Part model, mm, in its own coordinate system. Round coordinates to 2 decimals unless told otherwise and drop trailing zeros. Loops run counter-clockwise (first coordinate to the right, second up) from the corner with the lowest first, then second, coordinate; pieces in that order, holes last.
(1) Flat gauge pins, fed straight in: pin 1 (0.8 mm diameter, centred on y = 1.5, z = -2.5, fed in from -X); pin 2 (1.8 mm diameter, centred on x = -43.25, z = -31.5, fed in from +Y). Where does each tip first touch, or does it go through?
(2) Probe probe 1 along Z at (x, y) = (22, 2.3); probe 2 along X at (y, z) = (1.9, -31.5); probe 3 along Z at (x, y) = (-41, 2.75). List the from-to ranges inside material, lowest first.
(3) Cut at B-B on z = -6.5. List the corners of the cut face in (x, y), then the cut area to 4 significant figures.
(4) Cut at C-C on y = 0.6. Count the separate pieces of the cut face and the enclosed holes in it, then the cut area to 3 significant figures.
(5) Cut at A-A on x = -43.25. List the corners of the cut face in (y, z).
from build123d import *

# Parameters (mm, degrees)
SKETCH1_W           = 94.5
SKETCH1_H           = 70
BOSS_EXTRUDE1_DEPTH = 3
SKETCH3_R           = 1.5
CUT_EXTRUDE2_DEPTH  = 59.877521177
FILLET2_R           = 3
SKETCH5_W           = 13
SKETCH5_H           = 24
CUT_EXTRUDE3_DEPTH  = 59.877521177
FILLET3_R           = 1
FILLET5_R           = 1.5
FILLET6_R           = 1.5
FILLET7_R           = 1.5
FILLET8_R           = 1.5
FILLET9_R           = 1.5
FILLET10_R          = 1.5
FILLET11_R          = 1.5
FILLET12_R          = 1.5


with BuildPart() as part:
    # Sketch1 → Boss-Extrude1 (new body)
    with BuildSketch(Plane(origin=(0, 0, 0), x_dir=(1, 0, 0), z_dir=(0, 1, 0))):
        Rectangle(SKETCH1_W, SKETCH1_H)
    extrude(amount=BOSS_EXTRUDE1_DEPTH)

    # Sketch3 → Cut-Extrude2 (cut, through all)
    with BuildSketch(Plane(origin=(0, 3, 0), x_dir=(1, 0, 0), z_dir=(0, 1, 0))):
        with Locations(Location((43.75, 31.5, 0), (0, 0, 270))):
            Circle(SKETCH3_R)
        with Locations(Location((-43.25, 31.5, 0), (0, 0, 270))):
            Circle(SKETCH3_R)
        with Locations(Location((-43.25, -31.5, 0), (0, 0, 270))):
            Circle(SKETCH3_R)
        with Locations(Location((43.75, -31.5, 0), (0, 0, 270))):
            Circle(SKETCH3_R)
    extrude(amount=-CUT_EXTRUDE2_DEPTH, mode=Mode.SUBTRACT)

    # Fillet2
    fillet2_edges = [part.edges().sort_by_distance(p)[0] for p in [
        (47.25, 1.5, 35),
        (-47.25, 1.5, 35),
        (-47.25, 1.5, -35),
        (47.25, 1.5, -35),
    ]]
    fillet(fillet2_edges, radius=FILLET2_R)

    # Sketch5 → Cut-Extrude3 (cut, through all)
    with BuildSketch(Plane(origin=(0, 3, 0), x_dir=(1, 0, 0), z_dir=(0, 1, 0))):
        with Locations((-40.75, -1)):
            Rectangle(SKETCH5_W, SKETCH5_H)
        Polygon((-25.25, 1.5), (-25.25, 4.5), (-22.25, 4.5), (-22.25, 1.5), (-19.25, 1.5), (-19.25, -1.5), (-22.25, -1.5), (-22.25, -4.5), (-25.25, -4.5), (-25.25, -1.5), (-28.25, -1.5), (-28.25, 1.5), align=None)
        Polygon((25.25, 1.5), (25.25, 4.5), (22.25, 4.5), (22.25, 1.5), (19.25, 1.5), (19.25, -1.5), (22.25, -1.5), (22.25, -4.5), (25.25, -4.5), (25.25, -1.5), (28.25, -1.5), (28.25, 1.5), align=None)
    extrude(amount=-CUT_EXTRUDE3_DEPTH, mode=Mode.SUBTRACT)

    # Fillet3
    fillet3_edges = [part.edges().sort_by_distance(p)[0] for p in [
        (-34.25, 1.5, 13),
        (-47.25, 1.5, 13),
        (-47.25, 1.5, -11),
        (-34.25, 1.5, -11),
    ]]
    fillet(fillet3_edges, radius=FILLET3_R)

    # Fillet5
    fillet5_edges = [part.edges().sort_by_distance(p)[0] for p in [
        (-25.25, 1.5, -4.5),
        (-22.25, 1.5, -4.5),
    ]]
    fillet(fillet5_edges, radius=FILLET5_R - 0.0001)  # a hair under: the kernel refuses the full size

    # Fillet6
    fillet6_edges = [part.edges().sort_by_distance(p)[0] for p in [
        (-28.25, 1.5, 1.5),
        (-28.25, 1.5, -1.5),
    ]]
    fillet(fillet6_edges, radius=FILLET6_R - 0.0001)  # a hair under: the kernel refuses the full size

    # Fillet7
    fillet7_edges = [part.edges().sort_by_distance(p)[0] for p in [
        (-19.25, 1.5, -1.5),
        (-19.25, 1.5, 1.5),
    ]]
    fillet(fillet7_edges, radius=FILLET7_R - 0.0001)  # a hair under: the kernel refuses the full size

    # Fillet8
    fillet8_edges = [part.edges().sort_by_distance(p)[0] for p in [
        (-22.25, 1.5, 4.5),
        (-25.25, 1.5, 4.5),
    ]]
    fillet(fillet8_edges, radius=FILLET8_R - 0.0001)  # a hair under: the kernel refuses the full size

    # Fillet9
    fillet9_edges = [part.edges().sort_by_distance(p)[0] for p in [
        (25.25, 1.5, -4.5),
        (22.25, 1.5, -4.5),
    ]]
    fillet(fillet9_edges, radius=FILLET9_R - 0.0001)  # a hair under: the kernel refuses the full size

    # Fillet10
    fillet10_edges = [part.edges().sort_by_distance(p)[0] for p in [
        (28.25, 1.5, -1.5),
        (28.25, 1.5, 1.5),
    ]]
    fillet(fillet10_edges, radius=FILLET10_R - 0.0001)  # a hair under: the kernel refuses the full size

    # Fillet11
    fillet11_edges = [part.edges().sort_by_distance(p)[0] for p in [
        (25.25, 1.5, 4.5),
        (22.25, 1.5, 4.5),
    ]]
    fillet(fillet11_edges, radius=FILLET11_R - 0.0001)  # a hair under: the kernel refuses the full size

    # Fillet12
    fillet12_edges = [part.edges().sort_by_distance(p)[0] for p in [
        (19.25, 1.5, 1.5),
        (19.25, 1.5, -1.5),
    ]]
    fillet(fillet12_edges, radius=FILLET12_R - 0.0001)  # a hair under: the kernel refuses the full size


solid = part.part
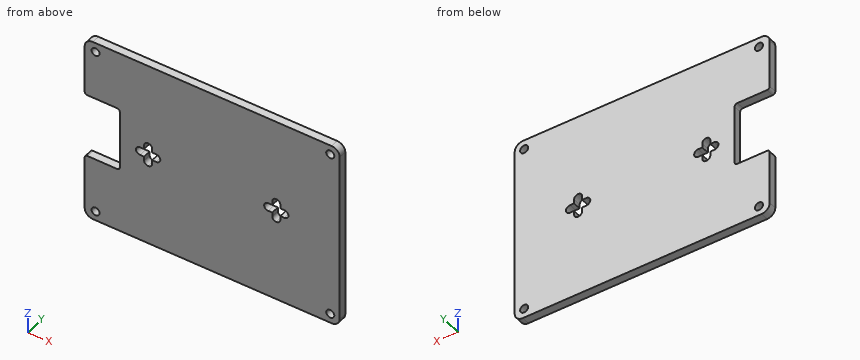
Final values:
1. pin 1: stops at x = -34.25
1. pin 2: passes through
2. probe 1: z = -35 to -1.5, 1.5 to 35
2. probe 2: x = -47.25 to -44.75, -41.75 to 42.25, 45.25 to 47.25
2. probe 3: z = -35 to -11, 13 to 35
3. outline: (-34.25, 0) - (47.25, 0) - (47.25, 3) - (-34.25, 3) - close
3. area: 244.5 mm2
4. separate pieces: 1
4. enclosed holes: 6
4. area: 6,180 mm2
5. outline: (0, -35) - (3, -35) - (3, -33) - (0, -33) - close; (0, -30) - (3, -30) - (3, -11) - (0, -11) - close; (0, 13) - (3, 13) - (3, 30) - (0, 30) - close; (0, 33) - (3, 33) - (3, 35) - (0, 35) - close
